Autodesk Fusion 360 part; units mm, degrees
sketch "Sketch1" plane through (0, 0, 0) normal (0, 0, 1) x (1, 0, 0)
  line L0 (0, 0) -> (60, 0)
  line L1 (60, 0) -> (60, 9)
  line L2 (60, 9) -> (0, 9)
  line L3 (0, 9) -> (0, 0)
  line L4 (12.5, 9) -> (47.5, 9)
  line L5 (47.5, 9) -> (47.5, 51)
  line L6 (47.5, 51) -> (12.5, 51)
  line L7 (12.5, 51) -> (12.5, 9)
  line L8 (30, 9) -> (30, 0) construction
  line L9 (30, 51) -> (30, 9) construction
  line L10 (14.5, 9) -> (14.5, 51)
  line L11 (45.5, 9) -> (45.5, 51)
  line L12 (16.5, 9) -> (16.5, 51)
  line L13 (43.5, 9) -> (43.5, 51)
  line L14 (20.75, 51) -> (39.25, 51)
  line L15 (39.25, 51) -> (39.25, 71)
  line L16 (39.25, 71) -> (20.75, 71)
  line L17 (20.75, 71) -> (20.75, 51)
  line L18 (35.25, 51) -> (35.25, 71)
  line L19 (24.75, 51) -> (24.75, 71)
  line L20 (14.5, 9) -> (46, 9)
  line L21 (46, 9) -> (46, 7)
  line L22 (46, 7) -> (14.5, 7)
  line L23 (14.5, 7) -> (14.5, 9)
  line L24 (39.25, 71) -> (47.5, 71)
  line L25 (47.5, 71) -> (47.5, 51)
  line L26 (47.5, 51) -> (39.25, 51)
  line L27 (39.25, 51) -> (39.25, 71)
  line L28 (20.75, 71) -> (12.5, 71)
  line L29 (12.5, 71) -> (12.5, 51)
  line L30 (12.5, 51) -> (20.75, 51)
  line L31 (20.75, 51) -> (20.75, 71)
  line L32 (47.5, 58.5) -> (12.5, 58.5)
  line L33 (12.5, 53) -> (47.5, 53)
  line L34 (47.5, 63.5) -> (12.5, 63.5)
  line L35 (12.5, 69) -> (47.5, 69)
  line L36 (46.5, 51) -> (46.5, 71)
  line L37 (13.5, 51) -> (13.5, 71)
  line L38 (47.5, 9) -> (47.5, 0) construction
  line L39 (12.5, 9) -> (12.5, 0) construction
  line L40 (60, 5) -> (0, 5) construction
  line L41 (20, 0) -> (40, 0)
  line L42 (40, 0) -> (40, 10.5)
  line L43 (40, 10.5) -> (20, 10.5)
  line L44 (20, 10.5) -> (20, 0)
  line L45 (12.5, 13.5) -> (47.5, 13.5)
  line L46 (47, 9) -> (47, 0) construction
  line L47 (13, 9) -> (13, 0) construction
  circle A0 centre (47, 5) radius 1.4
  circle A1 centre (13, 5) radius 1.4
  dimension "d1" = 60
  dimension "d2" = 9
  dimension "d3" = 35
  dimension "d4" = 42
  dimension "d8" = 2
  dimension "d9" = 2
  dimension "d10" = 4
  dimension "d11" = 4
  dimension "d27" = 18.5
  dimension "d28" = 20
  dimension "d29" = 9.25
  dimension "d34" = 4
  dimension "d35" = 4
  dimension "d45" = 2
  dimension "d49" = 1
  dimension "d50" = 1
  dimension "d51" = 5.5
  dimension "d52" = 2
  dimension "d53" = 5.5
  dimension "d54" = 2
  dimension "d66" = 5
  dimension "d74" = 20
  dimension "d75" = 10.5
  dimension "d76" = 10
  dimension "d80" = 4.5
  dimension "d82" = 34
  dimension "d83" = 17
  dimension "d84" = 2.8
  dimension "d85" = 2.8
extrude "Extrude1" add sketch "Sketch1" along normal blind 16 contours L0 L2 L3 L4 L22 L23 L44 | L0 L22 L41 L42 L44 | L0 L1 L2 L4 L21 L22 L42 | L2 L4 L20 L22 L42 L44 | L2 L4 L20 L22 L23 L44 | L2 L4 L20 L21 L22 L42
extrude "Extrude2" add sketch "Sketch1" along normal blind 2 contours L2 L4 L7 L10 L45 | L2 L4 L20 L42 L43 L44 | L2 L4 L12 L13 L20 L42 L43 L44 L45 | L2 L4 L10 L12 L20 L45 | L6 L7 L10 L30 L45 | L6 L10 L12 L30 L45 | L2 L4 L5 L11 L20 L45 | L2 L4 L11 L13 L20 L45 | L6 L12 L13 L14 L26 L30 L45 | L5 L6 L11 L26 L45 | L6 L11 L13 L26 L45
extrude "Extrude5" add sketch "Sketch1" along normal up to surface (16 mm away) contours L2 L4 L7 L10 L45 | L2 L4 L10 L12 L20 L45 | L6 L7 L10 L30 L45 | L6 L10 L12 L30 L45 | L2 L4 L5 L11 L20 L45 | L2 L4 L11 L13 L20 L45 | L5 L6 L11 L26 L45 | L6 L11 L13 L26 L45
extrude "Extrude6" cut sketch "Sketch1" along normal blind 2 from surface at 14 contours L6 L10 L12 L30 L45 | L6 L11 L13 L26 L45
extrude "Extrude7" add sketch "Sketch1" along normal blind 4 contours L6 L14 L17 L19 L31 L33 | L17 L19 L31 L32 L33 | L6 L14 L15 L18 L27 L33 | L6 L14 L18 L19 L33 | L17 L19 L31 L32 L34 | L18 L19 L32 L33 | L15 L18 L27 L32 L33 | L17 L19 L31 L34 L35 | L18 L19 L32 L34 | L15 L18 L27 L32 L34 | L16 L17 L19 L31 L35 | L18 L19 L34 L35 | L15 L18 L27 L34 L35 | L16 L18 L19 L35 | L15 L16 L18 L27 L35
extrude "Extrude8" add sketch "Sketch1" along normal blind 16 contours L6 L29 L30 L33 L37 | L6 L17 L30 L31 L33 L37 | L29 L32 L33 L37 | L17 L31 L32 L33 L37 | L29 L32 L34 L37 | L6 L25 L26 L33 L36 | L6 L15 L26 L27 L33 L36 | L6 L14 L17 L19 L31 L33 | L17 L19 L31 L32 L33 | L17 L31 L32 L34 L37 | L29 L34 L35 L37 | L25 L32 L33 L36 | L6 L14 L15 L18 L27 L33 | L17 L19 L31 L32 L34 | L17 L31 L34 L35 L37 | L28 L29 L35 L37 | L15 L27 L32 L33 L36 | L25 L32 L34 L36 | L15 L18 L27 L32 L33 | L17 L19 L31 L34 L35 | L17 L28 L31 L35 L37 | L15 L27 L32 L34 L36 | L25 L34 L35 L36 | L15 L18 L27 L32 L34 | L16 L17 L19 L31 L35 | L15 L27 L34 L35 L36 | L24 L25 L35 L36 | L15 L18 L27 L34 L35 | L15 L24 L27 L35 L36 | L15 L16 L18 L27 L35
extrude "Extrude10" cut sketch "Sketch1" along normal up to surface (16 mm away) contours L29 L32 L33 L37 | L29 L34 L35 L37 | L25 L32 L33 L36 | L25 L34 L35 L36
extrude "Extrude11" cut sketch "Sketch1" against normal blind 1 from surface at 16 contours L17 L31 L32 L33 L37 | L17 L19 L31 L32 L33 | L18 L19 L32 L33 | L17 L31 L34 L35 L37 | L15 L27 L32 L33 L36 | L15 L18 L27 L32 L33 | L17 L19 L31 L34 L35 | L18 L19 L34 L35 | L15 L27 L34 L35 L36 | L15 L18 L27 L34 L35
extrude "Extrude12" cut sketch "Sketch1" along normal blind 1 contours L17 L31 L32 L33 L37 | L17 L19 L31 L32 L33 | L18 L19 L32 L33 | L17 L31 L34 L35 L37 | L15 L27 L32 L33 L36 | L15 L18 L27 L32 L33 | L17 L19 L31 L34 L35 | L18 L19 L34 L35 | L15 L27 L34 L35 L36 | L15 L18 L27 L34 L35
extrude "Extrude13" cut sketch "Sketch1" along normal up to surface (16 mm away) contours A0 | A1
extrude "Extrude14" cut sketch "Sketch1" against normal blind 7 from surface at 16 contours L0 L22 L41 L42 L44 | L2 L4 L20 L22 L42 L44
fillet "Fillet3" radius 5.25 2 edges at (35.25, 61, 4) (24.75, 61, 4)
fillet "Fillet4" radius 2 2 edges at (43.5, 30, 2) (16.5, 30, 2)
fillet "Fillet4" radius 2 2 edges at (20, 4.5, 9) (40, 4.5, 9)
fillet "Fillet7" radius 2 10 edges at (24.75, 52, 16) (24.75, 55.75, 15) (24.75, 61, 16) (24.75, 66.25, 15) (24.75, 70, 16) (35.25, 70, 16) (35.25, 66.25, 15) (35.25, 61, 16) (35.25, 55.75, 15) (35.25, 52, 16)
fillet "Fillet7" radius 2 8 edges at (46.5, 55.75, 15) (46.5, 66.25, 15) (46.5, 55.75, 1) (46.5, 66.25, 1) (13.5, 55.75, 1) (13.5, 66.25, 1) (13.5, 66.25, 15) (13.5, 55.75, 15)
fillet "Fillet8" radius 2 2 edges at (12.5, 9, 8) (47.5, 9, 8)
chamfer "Chamfer1" distance 8.85 angle 45 2 edges at (60, 4.5, 0) (0, 4.5, 0)
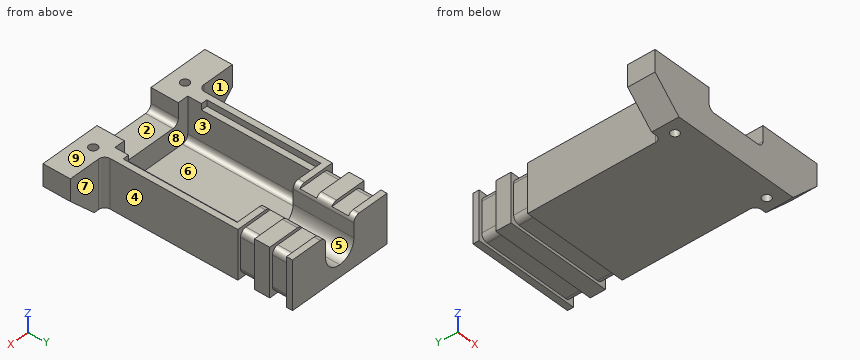
Can you work these out from the model? Positions are in its coordinate system, mm. Face numbers are marked on the shaded views. A direction names the side the tool comes from. Coordinates: 2 decimals unless noted, no trailing zeros. Loops run counter-clockwise (first coordinate to the right, second up) from the corner with the lowest first, then second, coordinate; pieces in that order, holes last. Notation, with made-up numbers: (40.5, -1.5) - (80.5, -1.5) arc R6 ccw to (80.5, 8.5) - close; hole circle Ø5 at (87, 3.5). An arc over 180 degrees is marked (long way). Answer as CSV lines item,"result". Start each with the question number.
1) Suppose I cut it at C-C (x = 7.5). Please give me the cut outline in (y, z), plus the area to 3 significant figures.
2) Suppose I cut it at B-B (y = 25). Please give me the cut outline in (x, z).
3) Which directions (+Z, -Z, +X, -X, +Y, -Y) give clear straight access to the entire face, cutting with the end or side of a thin tool? Please do the marked faces 1, 2, 3, 4 and 5.
4) I need wall thicknesses on line 1 (Y direction, x = 47, z = 4); line 2 (X direction, y = 6.5, z = 11); line 3 (X direction, y = 24.5, z = 4.25). Which ranges of each line are inside material? Lowest first, please. Write a range as from..to.
5) Thinking about a two-plate mould opening in Y: for the marked faces 6, 7, 8 and 9, which applies, pulls with the +Y half, pulls with the -Y half, needs draft (parallel to the pull), parting line crosses it, or undercut?
6) Suppose I cut it at A-A (y = 5). Please give me the cut outline in (x, z), plus the area to 3 significant figures.
7) For pin 1 (1 mm diameter, centred on y = 39, z = 6, fed in from -X); pin 2 (1 mm diameter, centred on x = 20.5, y = 11, fed in from +Z); pin 3 (6 mm diameter, centred on y = 55, z = 6, fed in from +X), each with a flat end and sliding along its axis, tell me the tip position at first contact or that it passes through.
Check result:
1,outline,"(0, 1.35) - (9, 1.35) - (9, 16) - (0, 16) - close"
1,area,"132 mm²"
2,outline,"(12.5, 0) - (47.5, 0) - (47.5, 16) - (45.5, 16) - (45.5, 14) - (43.5, 14) - (43.5, 4) arc R2 cw to (41.5, 2) - (18.5, 2) arc R2 cw to (16.5, 4) - (16.5, 14) - (14.5, 14) - (14.5, 16) - (12.5, 16) - close"
3,face 1,"+Z, -Z, -X, +Y"
3,face 2,"+Z, -Y"
3,face 3,"+Z"
3,face 4,"+Z, -Z, +X, +Y"
3,face 5,"+Z, +Y"
4,line 1,"y = 0..3.6, 6.4..53, 58.5..63.5, 69..71"
4,line 2,"x = 0..20, 40..60"
4,line 3,"x = 12.5..16.5, 43.5..47.5"
5,face 6,"undercut"
5,face 7,"pulls with the +Y half"
5,face 8,"undercut"
5,face 9,"needs draft"
6,outline,"(0, 8.85) - (8.85, 0) - (11.6, 0) - (11.6, 16) - (0, 16) - close; (14.4, 0) - (45.6, 0) - (45.6, 16) - (40, 16) - (40, 11) arc R2 cw to (38, 9) - (22, 9) arc R2 cw to (20, 11) - (20, 16) - (14.4, 16) - close; (48.4, 0) - (51.15, 0) - (60, 8.85) - (60, 16) - (48.4, 16) - close"
6,area,"654 mm²"
7,pin 1,"stops at x = 12.5"
7,pin 2,"stops at z = 2"
7,pin 3,"stops at x = 47.5"
